from build123d import *

# Parameters (mm, degrees)
F0_W      = 698.5
F0_H      = 355.6
F1_DEPTH  = 25.4
F2_W      = 88.9
F2_H      = 44.45
F3_DEPTH  = 3.175
F4_W      = 88.9
F4_H      = 44.45
F5_DEPTH  = 3.175
F6_W      = 88.9
F6_H      = 3.81
F7_DEPTH  = 3.175
F8_W      = 88.9
F8_H      = 3.81
F9_DEPTH  = 3.81
F11_DEPTH = 25.4
F12_W     = 101.6
F12_H     = 25.4
F13_DEPTH = 25.4
F14_R     = 25.39999


# Not quite as in the source:
# - a fillet or chamfer is up to 0.001 mm smaller than in the source, because OpenCascade refuses the exact size


with BuildPart() as f1:
    # F0 (on Top) → F1 (new body)
    with BuildSketch(Plane.XY):
        Rectangle(F0_W, F0_H)
    extrude(amount=F1_DEPTH)

    # F2 (on face) → F3 (cut)
    with BuildSketch(Plane.XY.offset(25.4)):
        with Locations((-254, 155.575)):
            Rectangle(F2_W, F2_H)
        with Locations((152.4, 155.575)):
            Rectangle(F2_W, F2_H)
    extrude(amount=-F3_DEPTH, mode=Mode.SUBTRACT)

    # F4 (on face) → F5 (cut)
    with BuildSketch(Plane(origin=(0, 0, 0), x_dir=(1, 0, 0), z_dir=(0, 0, -1))):
        with Locations((-254, 155.575)):
            Rectangle(F4_W, F4_H)
        with Locations((152.4, 155.575)):
            Rectangle(F4_W, F4_H)
    extrude(amount=-F5_DEPTH, mode=Mode.SUBTRACT)

    # F6 (on face) → F7 (cut)
    with BuildSketch(Plane.XY.offset(22.225)):
        with Locations((-254, 175.895)):
            Rectangle(F6_W, F6_H)
    extrude(amount=-F7_DEPTH, mode=Mode.SUBTRACT)

    # F8 (on face) → F9 (cut)
    with BuildSketch(Plane.XY.offset(22.225)):
        with Locations((152.4, 175.895)):
            Rectangle(F8_W, F8_H)
    extrude(amount=-F9_DEPTH, mode=Mode.SUBTRACT)

    # F10 (on face) → F11 (cut)
    with BuildSketch(Plane.XY.offset(25.4)):
        with BuildLine():
            Line((-311.0040204385, -12.7008390054), (-311.0040204385, -12.6991609946))
            ThreePointArc((-311.0040204385, -12.6991609946), (-298.45, 0), (-311.0040204385, 12.6991609946))
            Line((-311.0040204385, 12.6991609946), (-311.2959795615, 12.6991609946))
            Line((-311.2959795615, 12.6991609946), (-354.8822260717, 12.6991609946))
            Line((-354.8822260717, 12.6991609946), (-354.8822260717, -12.7008390054))
            Line((-354.8822260717, -12.7008390054), (-311.0040204385, -12.7008390054))
        make_face()
        with BuildLine():
            Line((-311.2959795615, 12.6991609946), (-311.0040204385, 12.6991609946))
            ThreePointArc((-311.0040204385, 12.6991609946), (-311.15, 12.7), (-311.2959795615, 12.6991609946))
        make_face()
        with BuildLine():
            Line((213.1756003467, 12.7013387805), (213.1756003467, 12.6986612195))
            ThreePointArc((213.1756003467, 12.6986612195), (200.66, 0), (213.1756003467, -12.6986612195))
            Line((213.1756003467, -12.6986612195), (213.5443996533, -12.6986612195))
            Line((213.5443996533, -12.6986612195), (264.16, -12.6986612195))
            ThreePointArc((264.16, -12.6986612195), (276.86, 0.0013387805), (264.16, 12.7013387805))
            Line((264.16, 12.7013387805), (213.1756003467, 12.7013387805))
        make_face()
        with BuildLine():
            Line((213.5443996533, -12.6986612195), (213.1756003467, -12.6986612195))
            ThreePointArc((213.1756003467, -12.6986612195), (213.36, -12.7), (213.5443996533, -12.6986612195))
        make_face()
    extrude(amount=-F11_DEPTH, mode=Mode.SUBTRACT)

    # F12 (on face) → F13 (cut)
    with BuildSketch(Plane.XY.offset(25.4)):
        with Locations((-44.45, -165.1)):
            Rectangle(F12_W, F12_H)
    extrude(amount=-F13_DEPTH, mode=Mode.SUBTRACT)

    # F14 (radius 25.4 in the source; OpenCascade refuses exactly that, so slightly less here)
    f14_edges = [f1.edges().sort_by_distance(p)[0] for p in [
        (-95.25, -152.4, 12.7),
        (6.35, -152.4, 12.7),
    ]]
    fillet(f14_edges, radius=F14_R)


solid = f1.part
Can you work these out from the model? Positions are in its coordinate system, mm. A direction names the side the tool comes from. Coordinates: 2 decimals unless noted, no trailing zeros. Write each loop counter-clockwise with the first axis right and the second up, starting at its lowest first coordinate (ties: lowest second). Pieces come first, ordered by that corner, then holes. Notation, with made-up numbers: (9.5, 51.5) - (67.5, 51.5) arc R21 ccw to (67.5, 76.5) - close; hole circle Ø11 at (39.25, -32.5). An arc over 180 degrees is marked (long way). Return JSON: item names as keys, results as strings. Group by question number.
Item 1: Please list where these lines run through material, in increasing order: probe 1 along Y at (x, z) = (264, 2); probe 2 along Y at (x, z) = (108.5, 2); probe 3 along X at (y, z) = (-5, 17.25).
Item 2: We'd pull the mould along X, two halves only. Please class faces 5 (the face through (-255, -156, 3.175)), 6 (the face through (-349.25, 94, 13)), 7 (the face through (276.857, -0.278, 12.878)), 8 (the face through (-5, 177.8, 13)): pulls with the +X half, pulls with the -X half, needs draft (parallel to the pull), parting line crosses it, or undercut.
Item 3: If we section it at C-C (y = 145): Write out the boundary of the cut face in (x, z) (3 decimals).
Item 4: I'm going to push flat-ended pins straight in: pin 1 Ø3 at (x, y) = (130.5, 176) entering from +Z (3 decimals); pin 2 Ø22 at (x, y) = (131.5, -165) entering from -Z (3 decimals); pin 3 Ø1 at (x, y) = (2.5, -75.5) entering from -Z. Where does each tip first touch, or does it pass through?
Item 5: Which directions (+Z, -Z, +X, -X, +Y, -Y) give clear straight access to the entire face, cutting with the end or side of a thin tool? Please do faces 1 (the face through (-87.61, -159.64, 12.52)), 2 (the face through (152, 154, 22.225)), 3 (the face through (238, -12.699, 13)), 4 (the face through (-330, -12.701, 13)).
Item 6: If we section it at A-A (x = 254): Write out the boundary of the cut face in (y, z), then the cut area to 3 significant figures.
Item 7: If we section it at B-B (y = 0): Write out the boundary of the cut face in (x, z), then the cut area to 3 significant figures.
Return value:
{
 "1": {"probe 1": "y = -177.8 to -12.7, 12.7 to 177.8", "probe 2": "y = -133.35 to 177.8", "probe 3": "x = -299.48 to 201.69, 275.83 to 349.25"},
 "2": {"face 5": "undercut", "face 6": "pulls with the -X half", "face 7": "undercut", "face 8": "needs draft"},
 "3": {"outline": "(-349.25, 0) - (349.25, 0) - (349.25, 25.4) - (196.85, 25.4) - (196.85, 22.225) - (107.95, 22.225) - (107.95, 25.4) - (-209.55, 25.4) - (-209.55, 22.225) - (-298.45, 22.225) - (-298.45, 25.4) - (-349.25, 25.4) - close"},
 "4": {"pin 1": "stops at z = 18.415", "pin 2": "stops at z = 3.175", "pin 3": "stops at z = 0"},
 "5": {"face 1": "+Z, -Z, -Y", "face 2": "+Z, +Y", "face 3": "+Z, -Z", "face 4": "+Z, -Z, -X"},
 "6": {"outline": "(-177.8, 0) - (-12.7, 0) - (-12.7, 25.4) - (-177.8, 25.4) - close; (12.7, 0) - (177.8, 0) - (177.8, 25.4) - (12.7, 25.4) - close", "area": "8,390 mm^2"},
 "7": {"outline": "(-298.45, 0) - (200.66, 0) - (200.66, 25.4) - (-298.45, 25.4) - close; (276.86, 0) - (349.25, 0) - (349.25, 25.4) - (276.86, 25.4) - close", "area": "14,500 mm^2"}
}
